The model under review builds one solid part; all positions refer to its coordinate system, in mm. Face numbers are marked on the shaded views. A direction names the side the tool comes from. Give positions to 0.01 mm unless a question says otherwise; leave off trailing zeros. Loops run counter-clockwise (first coordinate to the right, second up) from the corner with the lowest first, then second, coordinate; pieces in that order, holes last. Notation, with made-up numbers: (-21, -25.75) -> (-17, -25.75) arc R22 ccw to (-17, -6.75) -> close; hole circle Ø1 at (22, 79.25). An arc over 180 degrees is marked (long way). Write each question's results on one line, items separated by ' | '. Start each with the question number.
Q1. We need section A-A (x = -6). Write out the cut boundary in (y, z), plus the area to 3 significant figures.
Q2. Wall thickness on L1, parallel to X at y = 0.7, z = -4.5; L2, parallel to Z at x = -6, y = 0.35; L3, parallel to Z at x = -4.25, y = 0.7: over which ranges is each line inside the solid? List them lowest first. Write a range as [from, to].
Q3. We need section C-C (y = 0.85). Write out the cut boundary in (x, z), plus the area to 3 significant figures.
Q4. Mouldability with a two-part tool opening along Z and no side actions: class the marked faces 3, 4 and 5 as released by +Z, released by -Z, zero draft, split by the parting line, or undercut.
Q5. We need section B-B (y = 0.2). Write out the cut boundary in (x, z).
Q6. Insertion check: pin 1 Ø1 at (y, z) = (0.5, -6.5) entering from -X; pin 2 Ø1 at (x, y) = (-1.5, 1.5) entering from -Z. Each pin has a flat end and moves straight along its axis. Give the tip position at first contact, or say it passes through.
Q7. Machinability: for the marked faces 1 and 2, which of the approach directions +Z, -Z, +X, -X, +Y, -Y give a long, thin tool a straight path to every point of the face, cutting with its end or side? Answer none if there is none.
from build123d import *

# Parameters (mm, degrees)
SKETCH2_W           = 8
SKETCH2_H           = 2
BOSS_EXTRUDE1_DEPTH = 2
CUT_EXTRUDE1_DEPTH  = 12
CUT_EXTRUDE3_DEPTH  = 12


with BuildPart() as part:
    # Sketch2 → Boss-Extrude1 (new body)
    with BuildSketch(Plane(origin=(0, 0, 0), x_dir=(1, 0, 0), z_dir=(0, 1, 0))):
        Polygon((3.177780174, 7.609317523), (1.977355898, -0.300106069), (0, 0), (1.200424276, 7.909423592), align=None)
        Polygon((1.977355898, -0.300106069), (0, -2), (0, 0), align=None)
        with Locations((-4, -1)):
            Rectangle(SKETCH2_W, SKETCH2_H)
    extrude(amount=BOSS_EXTRUDE1_DEPTH)

    # Sketch3 → Cut-Extrude1 (cut)
    with BuildSketch(Plane.ZY.offset(8)):
        with BuildLine():
            ThreePointArc((1.5, 1), (1.353553391, 1.353553391), (1, 1.5))
            Line((1, 1.5), (1, 0.5))
            ThreePointArc((1, 0.5), (1.353553391, 0.646446609), (1.5, 1))
        make_face()
        with BuildLine():
            Line((1, 0.5), (1, 1.5))
            ThreePointArc((1, 1.5), (0.646446609, 1.353553391), (0.5, 1))
            ThreePointArc((0.5, 1), (0.646446609, 0.646446609), (1, 0.5))
        make_face()
    extrude(amount=-CUT_EXTRUDE1_DEPTH, mode=Mode.SUBTRACT)

    # Sketch4 → Cut-Extrude3 (cut)
    with BuildSketch(Plane(origin=(1.200424276, 0, -7.909423592), x_dir=(-0.988677949, 0, -0.150053035), z_dir=(0.150053035, 0, -0.988677949))):
        with BuildLine():
            ThreePointArc((-0.5, 1), (-0.646446609, 1.353553391), (-1, 1.5))
            Line((-1, 1.5), (-1, 0.5))
            ThreePointArc((-1, 0.5), (-0.646446609, 0.646446609), (-0.5, 1))
        make_face()
        with BuildLine():
            Line((-1, 0.5), (-1, 1.5))
            ThreePointArc((-1, 1.5), (-1.353553391, 1.353553391), (-1.5, 1))
            ThreePointArc((-1.5, 1), (-1.353553391, 0.646446609), (-1, 0.5))
        make_face()
    extrude(amount=-CUT_EXTRUDE3_DEPTH, mode=Mode.SUBTRACT)


solid = part.part
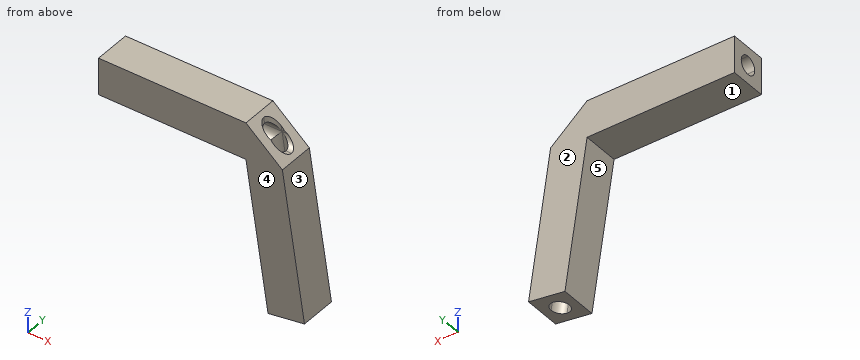
Output:
1) outline: (0, 0) -> (2, 0) -> (2, 2) -> (0, 2) -> close; hole circle Ø1 at (1, 1) | area: 3.21 mm2
2) L1: [0.68, 1.29], [2.1, 2.71] | L2: [0, 2] | L3: [0, 0.6], [1.4, 2]
3) outline: (-8, 0) -> (0, 0) -> (1.2, -7.91) -> (1.72, -7.83) -> (0.45, 0.52) -> (-8, 0.52) -> close; (-8, 1.48) -> (0.3, 1.48) -> (0.26, 1.78) -> (0, 2) -> (-8, 2) -> close; (1.41, 0.52) -> (2.66, -7.69) -> (3.18, -7.61) -> (1.98, 0.3) -> (1.72, 0.52) -> close | area: 17.2 mm2
4) face 3: released by +Z | face 4: zero draft | face 5: released by -Z
5) outline: (-8, 0) -> (0, 0) -> (1.2, -7.91) -> (3.18, -7.61) -> (1.98, 0.3) -> (0, 2) -> (-8, 2) -> close
6) pin 1: x = 0.91 | pin 2: z = 0
7) face 1: -Z, -X, +Y, -Y | face 2: +Z, -Z, +X, -X, +Y
